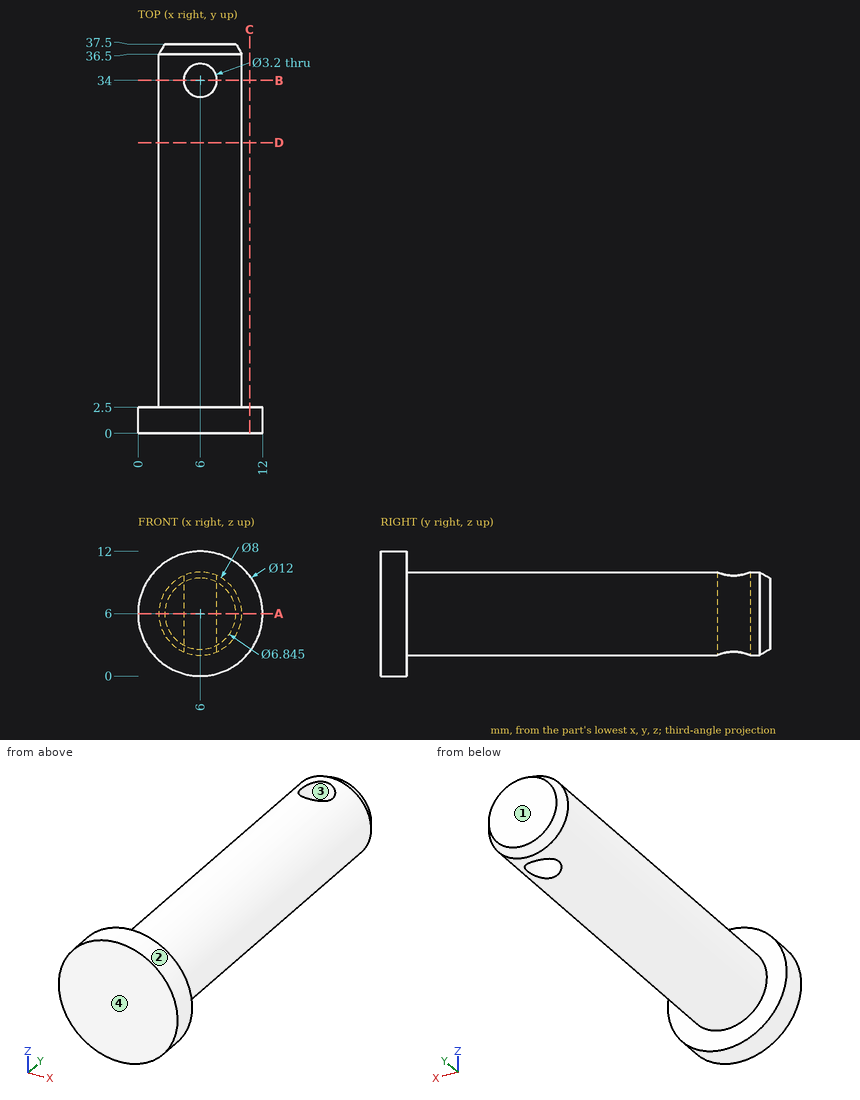
Study the drawing (mm; zero at the part's minimum x, y, z) and answer. Coordinates: 2 decimals unless noted, no trailing zeros. Loops run counter-clockwise (first coordinate to the right, second up) from the corner with the lowest first, then second, coordinate; pieces in that order, holes last. Notation, with made-up numbers: (55.25, 87) -> (91.25, 87) arc R12 ccw to (91.25, 108) -> close; hole circle Ø6 at (72.5, 43). An arc over 180 degrees is marked (long way). Answer in a Markdown table with one row per item. Add a question column.
1. Determine the mould class of the marked faces 1, 2, 3 and 4 for opening direction Y: +Y half, -Y half, draft (parallel to the pull), parting line (faces both ways), or undercut.
2. Consider line 1 (Y direction, x = 6, z = 4.5); line 2 (X direction, y = 34, z = 7); line 3 (X direction, y = 34.5, z = 7.5). Determine where each line is inside the solid, lowest interval first. Write a range as [from, to].
3. Flat-ended cylindrical pins translate along their axes: P1, Ø5, axis at x = 4, y = 27.5, coming from the -Z side; P2, Ø4, axis at x = 6, y = 34, coming from the +Z side; P3, Ø4, axis at x = 11, y = 23.5, coming from the +Z side (1 decimal). Find the tip coordinate at first contact, or state that the pin passes through.
4. The part is cut by section D-D, the plane y = 28. Write down the section's boundary in (x, z), then the cut area to 3 significant figures.
5. The part is cut by section C-C, the plane x = 10.75. Write down the section's boundary in (y, z).
6. The part is cut by section B-B, the plane y = 34. Write down the section's boundary in (x, z).
7. The part is cut by section A-A, the plane z = 6. Write down the section's boundary in (x, y), then the cut area to 3 significant figures.
Answer below:
| question | item | result |
|---|---|---|
| 1 | face 1 | +Y half |
| 1 | face 2 | draft |
| 1 | face 3 | undercut |
| 1 | face 4 | -Y half |
| 2 | line 1 | [0, 32.4], [35.6, 37.5] |
| 2 | line 2 | [2.13, 4.4], [7.6, 9.87] |
| 2 | line 3 | [2.29, 4.48], [7.52, 9.71] |
| 3 | P1 | z = 2 |
| 3 | P2 | z = 10 |
| 3 | P3 | z = 8.6 |
| 4 | outline | circle Ø8 at (6, 6) |
| 4 | area | 50.3 mm2 |
| 5 | outline | (0, 2.33) -> (2.5, 2.33) -> (2.5, 9.67) -> (0, 9.67) -> close |
| 6 | outline | (4.4, 2.33) -> (4.4, 9.67) arc R4 ccw to start; (7.6, 2.33) arc R4 ccw to (7.6, 9.67) -> close |
| 7 | outline | (0, 0) -> (12, 0) -> (12, 2.5) -> (10, 2.5) -> (10, 36.5) -> (9.42, 37.5) -> (2.58, 37.5) -> (2, 36.5) -> (2, 2.5) -> (0, 2.5) -> close; hole circle Ø3.2 at (6, 34) |
| 7 | area | 301 mm2 |
